Read the model definition and answer for the solid it produces. Units are mm, in the model's axes. A direction names the side the tool comes from. Give positions to 0.01 mm unless a question says otherwise; leave off trailing zeros. Answer as CSV lines item,"result". Start each with the question number.
1) Flat-ended cylindrical pins translate along their axes: pin 1 Ø0.8 at (x, z) = (19.5, 4) entering from +Y; pin 2 Ø1.5 at (y, z) = (-14.5, 2.5) entering from +X; pin 3 Ø8 at (x, y) = (14.5, -22.5) entering from +Z. Find the tip coordinate at first contact, or state that the pin passes through.
2) Straight lines are drawn through the part: L1, parallel to X at y = -59, z = 5; L2, parallel to X at y = -58.5, z = 2.5; L3, parallel to Z at x = -25, y = -27.5. For each, find the intervals that lie inside material, in ascending order. Write a range as from..to.
3) For faces 1 (the face through (-21.93, -32.75, 3.18)), 2 (the face through (21.049, -32.707, 5.819)), 3 (the face through (-9.36, -54.8, 5.82)), 4 (the face through (9.611, -55.664, 3.182)), 5 (the face through (-15.086, -51.059, 0.581)), determine the directions among +Z, -Z, +X, -X, +Y, -Y from which every point of the face is accessible in a straight line to the end or side of a thin tool.
4) The mould has two halves that part along X. Classify faces 6 (the face through (21.66, -32.944, 3.182)), 7 (the face through (9.6, -55, 0.6)), 8 (the face through (20, -25.763, 3)): +X half, -X half, draft (parallel to the pull), parting line (faces both ways), or undercut.
```python
from build123d import *

# Parameters (mm, degrees)
F1_DEPTH    = 6.4
F5_R        = 1.9313708499
F6_T1_DEPTH = 6.4
F6_T4_ANGLE = 144
F6_T6_ANGLE = 144


# Not quite as in the source:
# - a fillet or chamfer that OpenCascade refuses, or shapes differently, is made with other operations: its cross-section is extruded or revolved along the edge and cut away or added


with BuildPart() as f1:
    # F0 (on Top) → F1 (new body)
    with BuildSketch(Plane.XY):
        Polygon((-31.5438667271, -25.7632551613), (-12.0486849532, -39.9273338113), (-19.495181774, -62.8452944863), (0, -48.6812158363), (19.495181774, -62.8452944863), (12.0486849532, -39.9273338113), (31.5438667271, -25.7632551613), (7.4464968208, -25.7632551613), (0, -2.8452944863), (-7.4464968208, -25.7632551613), align=None)
    extrude(amount=F1_DEPTH)

    # F5
    f5_edges = [f1.edges().sort_by_distance(p)[0] for p in [
        (-21.796276, -32.845294, 6.4),
        (-15.771933, -51.386314, 6.4),
        (-9.747591, -55.763255, 6.4),
        (9.747591, -55.763255, 6.4),
        (15.771933, -51.386314, 6.4),
        (21.796276, -32.845294, 6.4),
        (19.495182, -25.763255, 6.4),
        (3.723248, -14.304275, 6.4),
        (-3.723248, -14.304275, 6.4),
        (-19.495182, -25.763255, 6.4),
        (-21.796276, -32.845294, 0),
        (-15.771933, -51.386314, 0),
        (-9.747591, -55.763255, 0),
        (9.747591, -55.763255, 0),
        (15.771933, -51.386314, 0),
        (21.796276, -32.845294, 0),
        (19.495182, -25.763255, 0),
        (3.723248, -14.304275, 0),
        (-3.723248, -14.304275, 0),
        (-19.495182, -25.763255, 0),
    ]]
    fillet(f5_edges, radius=F5_R)

    # F6: fillet of radius 2.5491174943 on 1 edges, made by hand

    # F6_s2 → F6_t1 (cut)
    with BuildSketch(Plane.XY):
        with BuildLine():
            ThreePointArc((2.4243548038, -10.3066913542), (0, -8.5452944863), (-2.4243548038, -10.3066913542))
            Line((-2.4243548038, -10.3066913542), (0, -2.8452944863))
            Line((0, -2.8452944863), (2.4243548038, -10.3066913542))
        make_face()
    extrude(amount=F6_T1_DEPTH, mode=Mode.SUBTRACT)

    # F6_s3 → F6_t4 (revolve, cut)
    with BuildSketch(Plane(origin=(-3.2605658725, -10.0349899078, 0), x_dir=(0, 0, 1), z_dir=(-0.3090169944, -0.9510565163, 0))):
        with BuildLine():
            ThreePointArc((0, -2.8106152002), (0.5656854249, -1.4449297752), (1.9313708499, -0.8792443503))
            Line((1.9313708499, -0.8792443503), (0, -0.8792443503))
            Line((0, -0.8792443503), (0, -2.8106152002))
        make_face()
    revolve(axis=Axis((0, -11.0944119806, 0), (0, 0, -1)), revolution_arc=F6_T4_ANGLE, mode=Mode.SUBTRACT)

    # F6_s5 → F6_t6 (revolve, cut)
    with BuildSketch(Plane(origin=(3.2605658725, -10.0349899078, 0), x_dir=(0, 0, 1), z_dir=(0.3090169944, -0.9510565163, 0))):
        with BuildLine():
            ThreePointArc((6.4, 2.8106152002), (5.8343145751, 1.4449297752), (4.4686291501, 0.8792443503))
            Line((4.4686291501, 0.8792443503), (6.4, 0.8792443503))
            Line((6.4, 0.8792443503), (6.4, 2.8106152002))
        make_face()
    revolve(axis=Axis((0, -11.0944119806, 6.4), (0, 0, 1)), revolution_arc=F6_T6_ANGLE, mode=Mode.SUBTRACT)


solid = f1.part
```
Findings below:
1,pin 1,"y = -25.76"
1,pin 2,"x = 4.03"
1,pin 3,"z = 5.99"
2,L1,"-18.17..-14.33, 14.33..18.17"
2,L2,"-18.08..-13.51, 13.51..18.08"
2,L3,"0.01..6.39"
3,face 1,"+Z, -Z, -X"
3,face 2,"+Z, +X"
3,face 3,"+Z, -Y"
3,face 4,"+Z, -Z, -Y"
3,face 5,"-Z, -X"
4,face 6,"+X half"
4,face 7,"undercut"
4,face 8,"draft"
